Geometry check sheet. Reference: the model listing, model coordinates, mm. A direction names the side the tool comes from. Round coordinates to 2 decimals unless told otherwise and drop trailing zeros. Write each loop counter-clockwise with the first axis right and the second up, starting at its lowest first coordinate (ties: lowest second). Pieces come first, ordered by that corner, then holes. Notation, with made-up numbers: (28.25, -8) - (78.25, -8) arc R22 cw to (78.25, 23) - close; hole circle Ø8 at (0.25, 11.5). An arc over 180 degrees is marked (long way). Return JSON: item names as keys, results as strings.
```python
from build123d import *

# Parameters (mm, degrees)
PAD_DEPTH       = 40
SKETCH001_R     = 13
POCKET_DEPTH    = 37
SKETCH002_W     = 15
SKETCH002_H     = 20
POCKET001_DEPTH = 37
SKETCH003_R     = 5.5
POCKET002_DEPTH = 2.5


with BuildPart() as part:
    # Sketch → Pad (new body)
    with BuildSketch(Plane.XY):
        with BuildLine():
            ThreePointArc((13.5, 0), (-9.545941, 9.545942), (0, -13.5))
            ThreePointArc((0, -13.5), (-9.545941, -36.545942), (13.5, -27))
            ThreePointArc((13.5, -27), (27, -40.5), (40.5, -27))
            ThreePointArc((40.5, -27), (63.545941, -36.545942), (54, -13.5))
            ThreePointArc((54, -13.5), (63.545941, 9.545942), (40.5, 0))
            ThreePointArc((40.5, 0), (27, 13.5), (13.5, 0))
        make_face()
    extrude(amount=PAD_DEPTH)

    # Sketch001 (on Face8 of Pad) → Pocket (cut)
    with BuildSketch(Plane.XY.offset(40)):
        Circle(SKETCH001_R)
        with Locations((0, -27)):
            Circle(SKETCH001_R)
        with Locations((27, 0)):
            Circle(SKETCH001_R)
        with Locations((27, -27)):
            Circle(SKETCH001_R)
        with Locations((54, 0)):
            Circle(SKETCH001_R)
        with Locations((54, -27)):
            Circle(SKETCH001_R)
    extrude(amount=-POCKET_DEPTH, mode=Mode.SUBTRACT)

    # Sketch002 (on Face5 of Pocket) → Pocket001 (cut)
    with BuildSketch(Plane.XY.offset(40)):
        with Locations((0, 10)):
            Rectangle(SKETCH002_W, SKETCH002_H)
        with Locations((0, -35)):
            Rectangle(SKETCH002_W, SKETCH002_H)
        with Locations((27.5, 10)):
            Rectangle(SKETCH002_W, SKETCH002_H)
        with Locations((55, 10)):
            Rectangle(SKETCH002_W, SKETCH002_H)
        with Locations((27.5, -35)):
            Rectangle(SKETCH002_W, SKETCH002_H)
        with Locations((55, -35)):
            Rectangle(SKETCH002_W, SKETCH002_H)
    extrude(amount=-POCKET001_DEPTH, mode=Mode.SUBTRACT)

    # Sketch003 (on Face2 of Pocket001) → Pocket002 (cut)
    with BuildSketch(Plane(origin=(0, 0, 0), x_dir=(1, 0, 0), z_dir=(0, 0, -1))):
        with Locations((12, 13.5)):
            Circle(SKETCH003_R)
        with Locations((27, 13.5)):
            Circle(SKETCH003_R)
        with Locations((42, 13.5)):
            Circle(SKETCH003_R)
    extrude(amount=-POCKET002_DEPTH, mode=Mode.SUBTRACT)


solid = part.part
```
(1) Section check A-A, the plane x = -4. Enter the section's corners in (y, z).
Response values:
{"outline": "(-39.89, 0) - (-14.11, 0) - (-14.11, 40) - (-14.63, 40) - (-14.63, 3) - (-39.89, 3) - close; (-12.89, 0) - (12.89, 0) - (12.89, 3) - (-12.37, 3) - (-12.37, 40) - (-12.89, 40) - close"}
(2) Gauge pin test, flat ends, axial feed: pin 1 (15.5 mm diameter, centred on x = 27, y = -27, fed in from +Z); pin 2 (12 mm diameter, centred on y = -28, z = 26.5, fed in from +X); pin 3 (0.7 mm diameter, centred on y = 11, z = 16.5, fed in from -X); pin 4 (8 mm diameter, centred on x = 14.5, z = 23.5, fed in from -Y). Record the tip position at first contact, or that the pin passes through.
Response values:
{"pin 1": "stops at z = 3", "pin 2": "stops at x = 67.5", "pin 3": "stops at x = -8.3", "pin 4": "stops at y = -37.49"}
(3) Access from +Z, -Z, +X, -X, +Y, -Y to the whole of each face (thin tool, end or side, straight path). Record for faces 1 (the face through (37.6, -10.2, 1.2)), 2 (the face through (25.929, -12.956, 21.759)).
Response values:
{"face 1": "-Z", "face 2": "+Z"}
(4) Section check C-C, the plane x = 27. Enter the section's corners in (y, z), plus the area to 4 significant figures.
Response values:
{"outline": "(-40.5, 0) - (-19, 0) - (-19, 2.5) - (-8, 2.5) - (-8, 0) - (13.5, 0) - (13.5, 3) - (-13, 3) - (-13, 40) - (-14, 40) - (-14, 3) - (-40.5, 3) - close", "area": "171.5 mm^2"}
(5) Material ranges on line 1 along Y through (x, z) = (37.5, 38); line 2 along X through (y, z) = (-19, 27.5); line 3 along X through (y, z) = (-4, 9), recorded low to high. Write a range as [from, to].
Response values:
{"line 1": "y = [-35.49, -34.66], [-19.34, -7.66], [7.66, 8.49]", "line 2": "x = [-10.87, -10.25], [10.25, 16.75], [37.25, 43.75], [64.25, 64.87]", "line 3": "x = [-12.89, -12.37], [12.37, 14.63], [39.37, 41.63], [66.37, 66.89]"}
(6) Section check B-B, the plane y = -28.5. Enter the section's corners in (x, z).
Response values:
{"outline": "(-13.42, 0) - (13.42, 0) - (13.42, 40) - (12.91, 40) - (12.91, 3) - (-12.91, 3) - (-12.91, 40) - (-13.42, 40) - close; (13.58, 0) - (40.42, 0) - (40.42, 40) - (39.91, 40) - (39.91, 3) - (14.09, 3) - (14.09, 40) - (13.58, 40) - close; (40.58, 0) - (67.42, 0) - (67.42, 40) - (66.91, 40) - (66.91, 3) - (41.09, 3) - (41.09, 40) - (40.58, 40) - close"}
